Can you work these out from the model? Positions are in its coordinate system, mm. Face numbers are marked on the shaded views. A direction names the side the tool comes from. Round coordinates to 2 decimals unless told otherwise and drop trailing zeros. Loops run counter-clockwise (first coordinate to the right, second up) from the corner with the lowest first, then second, coordinate; pieces in that order, holes last. Notation, with made-up numbers: (52, 0.25) -> (92, 0.25) arc R27 cw to (92, 30.25) -> close; hole circle Ø2 at (81, 80.25). An arc over 180 degrees is marked (long way). Use a Markdown table: item, result.
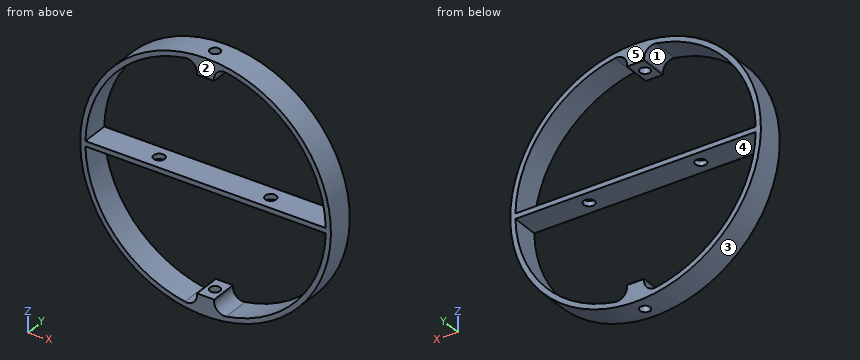
from build123d import *

# Parameters (mm, degrees)
ESQUISSE1_R             = 36.5
ESQUISSE1_R_2           = 35
BOSS_EXTRU_1_DEPTH      = 4
ENL_V_MAT_EXTRU_1_REACH = 83.714
ESQUISSE3_R             = 1.5
ENL_V_MAT_EXTRU_2_REACH = 54.305
ESQUISSE2_R             = 1.6
CONG_1_R                = 3


with BuildPart() as part:
    # Esquisse1 → Boss.-Extru.1 (new, symmetric)
    # profile 1 of 7: a face of its own
    with BuildSketch(Plane(origin=(0, 0, 0), x_dir=(1, 0, 0), z_dir=(0, 1, 0))):
        with Locations(Location((0, 0, 0), (0, 0, 270))):
            Circle(ESQUISSE1_R)
        Circle(ESQUISSE1_R_2, mode=Mode.SUBTRACT)
    # profile 2 of 7: a face of its own
    with BuildSketch(Plane(origin=(0, 0, 0), x_dir=(1, 0, 0), z_dir=(0, 1, 0))):
        with BuildLine():
            Line((34.991963363, 0.75), (0, 0.75))
            Line((0, 0.75), (0, -0.75))
            Line((0, -0.75), (34.991963363, -0.75))
            ThreePointArc((34.991963363, -0.75), (34.997990783, -0.375021529), (35, 0))
            ThreePointArc((35, 0), (34.997990783, 0.375021529), (34.991963363, 0.75))
        make_face()
    # profile 3 of 7: a face of its own
    with BuildSketch(Plane(origin=(0, 0, 0), x_dir=(1, 0, 0), z_dir=(0, 1, 0))):
        with BuildLine():
            Line((0, 0.75), (-34.991963363, 0.75))
            ThreePointArc((-34.991963363, 0.75), (-35, 0), (-34.991963363, -0.75))
            Line((-34.991963363, -0.75), (0, -0.75))
            Line((0, -0.75), (0, 0.75))
        make_face()
    # profile 4 of 7: a face of its own
    with BuildSketch(Plane(origin=(0, 0, 0), x_dir=(1, 0, 0), z_dir=(0, 1, 0))):
        with BuildLine():
            Line((0, 0.75), (-34.991963363, 0.75))
            ThreePointArc((-34.991963363, 0.75), (-35, 0), (-34.991963363, -0.75))
            Line((-34.991963363, -0.75), (0, -0.75))
            Line((0, -0.75), (0, 0.75))
        make_face()
    # profile 5 of 7: a face of its own
    with BuildSketch(Plane(origin=(0, 0, 0), x_dir=(1, 0, 0), z_dir=(0, 1, 0))):
        with BuildLine():
            Line((34.991963363, 0.75), (0, 0.75))
            Line((0, 0.75), (0, -0.75))
            Line((0, -0.75), (34.991963363, -0.75))
            ThreePointArc((34.991963363, -0.75), (34.997990783, -0.375021529), (35, 0))
            ThreePointArc((35, 0), (34.997990783, 0.375021529), (34.991963363, 0.75))
        make_face()
    # profile 6 of 7: a face of its own
    with BuildSketch(Plane(origin=(0, 0, 0), x_dir=(1, 0, 0), z_dir=(0, 1, 0))):
        with BuildLine():
            Line((-2.5, -30.910600109), (-2.5, -34.910600109))
            ThreePointArc((-2.5, -34.910600109), (0, -35), (2.5, -34.910600109))
            Line((2.5, -34.910600109), (2.5, -30.910600109))
            Line((2.5, -30.910600109), (-2.5, -30.910600109))
        make_face()
    # profile 7 of 7: a face of its own
    with BuildSketch(Plane(origin=(0, 0, 0), x_dir=(1, 0, 0), z_dir=(0, 1, 0))):
        with BuildLine():
            ThreePointArc((2.5, 34.910600109), (0, 35), (-2.5, 34.910600109))
            Line((-2.5, 34.910600109), (-2.5, 30.910600109))
            Line((-2.5, 30.910600109), (2.5, 30.910600109))
            Line((2.5, 30.910600109), (2.5, 34.910600109))
        make_face()
    extrude(amount=BOSS_EXTRU_1_DEPTH, both=True)

    # Esquisse3 → Enlèv. mat.-Extru.1 (cut, up to next)
    with BuildSketch(Plane.XY.offset(36.5), mode=Mode.PRIVATE) as enl_v_mat_extru_1_sk1:
        Circle(ESQUISSE3_R)
    enl_v_mat_extru_1_tool1 = extrude(enl_v_mat_extru_1_sk1.sketch, amount=-ENL_V_MAT_EXTRU_1_REACH, mode=Mode.PRIVATE) & part.part
    enl_v_mat_extru_1 = enl_v_mat_extru_1_tool1.solids().sort_by_distance((0, 0, 36.5))[0]
    add(enl_v_mat_extru_1, mode=Mode.SUBTRACT)

    # Symétrie1: Enlèv. mat.-Extru.1 across plane
    add(enl_v_mat_extru_1.mirror(Plane.XY), mode=Mode.SUBTRACT)

    # Esquisse2 → Enlèv. mat.-Extru.2 (cut, up to next)
    with BuildSketch(Plane.XY.offset(0.75), mode=Mode.PRIVATE) as enl_v_mat_extru_2_sk1:
        with Locations((-16.256, 0)):
            Circle(ESQUISSE2_R)
    enl_v_mat_extru_2_tool1 = extrude(enl_v_mat_extru_2_sk1.sketch, amount=-ENL_V_MAT_EXTRU_2_REACH, mode=Mode.PRIVATE) & part.part
    # Esquisse2 → Enlèv. mat.-Extru.2 (cut, up to next)
    with BuildSketch(Plane.XY.offset(0.75), mode=Mode.PRIVATE) as enl_v_mat_extru_2_sk2:
        with Locations((16.256, 0)):
            Circle(ESQUISSE2_R)
    enl_v_mat_extru_2_tool2 = extrude(enl_v_mat_extru_2_sk2.sketch, amount=-ENL_V_MAT_EXTRU_2_REACH, mode=Mode.PRIVATE) & part.part
    add(enl_v_mat_extru_2_tool1.solids().sort_by_distance((-16.256, 0, 0.75))[0], mode=Mode.SUBTRACT)
    add(enl_v_mat_extru_2_tool2.solids().sort_by_distance((16.256, 0, 0.75))[0], mode=Mode.SUBTRACT)

    # Congé1
    cong_1_edges = [part.edges().sort_by_distance(p)[0] for p in [
        (2.5, 0, -34.910600109),
        (-2.5, 0, -34.910600109),
        (-2.5, 0, 34.910600109),
        (2.5, 0, 34.910600109),
    ]]
    fillet(cong_1_edges, radius=CONG_1_R)


solid = part.part
1. If we mould it in two halves opening along Z, with no side actions, what happens to the marked faces 1, 2 and 3? For each: +Z half, -Z half, draft (parallel to the pull), parting line (faces both ways), or undercut.
Answer sheet:
| item | result |
|---|---|
| face 1 | undercut |
| face 2 | draft |
| face 3 | parting line |
2. I want a section at D-D (x = 13). Please give me the cut outline in (y, z), plus the area to 3 significant figures.
Answer sheet:
| item | result |
|---|---|
| outline | (-4, -34.11) -> (4, -34.11) -> (4, -32.5) -> (-4, -32.5) -> close; (-4, -0.75) -> (4, -0.75) -> (4, 0.75) -> (-4, 0.75) -> close; (-4, 32.5) -> (4, 32.5) -> (4, 34.11) -> (-4, 34.11) -> close |
| area | 37.8 mm² |
3. I need wall thicknesses on line 1 (Z direction, x = -27, y = -3.25); line 2 (Z direction, x = 16.5, y = -2); line 3 (Y direction, x = 0, z = 34.7). Which ranges of each line are inside material? Lowest first, please.
Answer sheet:
| item | result |
|---|---|
| line 1 | z = -24.56 to -22.27, -0.75 to 0.75, 22.27 to 24.56 |
| line 2 | z = -32.56 to -30.87, -0.75 to 0.75, 30.87 to 32.56 |
| line 3 | y = -4 to -1.5, 1.5 to 4 |
4. I want a section at B-B (y = 2.75). Please give me the cut outline in (x, z), plus the area to 3 significant figures.
Answer sheet:
| item | result |
|---|---|
| outline | circle Ø73 at (0, 0); hole (-34.99, -0.75) arc R35 ccw to (-6.02, -34.48) arc R3 ccw to (-2.5, -31.52) -> (-2.5, -30.91) -> (2.5, -30.91) -> (2.5, -31.52) arc R3 ccw to (6.02, -34.48) arc R35 ccw to (34.99, -0.75) -> close; hole (-34.99, 0.75) -> (34.99, 0.75) arc R35 ccw to (6.02, 34.48) arc R3 ccw to (2.5, 31.52) -> (2.5, 30.91) -> (-2.5, 30.91) -> (-2.5, 31.52) arc R3 ccw to (-6.02, 34.48) arc R35 ccw to start |
| area | 493 mm² |
5. Will these pins go through, and if not, where does the flat tip stop? pin 1 Ø3.5 at (x, y) = (16.256, 0) entering from -Z; pin 2 Ø2.5 at (x, y) = (0, 0) entering from -Z; pin 3 Ø0.7 at (y, z) = (2, 31.5) entering from -X; pin 4 Ø4 at (x, y) = (0, 0) entering from -Z.
Answer sheet:
| item | result |
|---|---|
| pin 1 | stops at z = -33.49 |
| pin 2 | stops at z = -0.75 |
| pin 3 | stops at x = -19.02 |
| pin 4 | stops at z = -36.5 |
6. I want a section at C-C (z = 4.5). Please give me the cut outline in (x, y), plus the area to 3 significant figures.
Answer sheet:
| item | result |
|---|---|
| outline | (-36.22, -4) -> (-34.71, -4) -> (-34.71, 4) -> (-36.22, 4) -> close; (34.71, -4) -> (36.22, -4) -> (36.22, 4) -> (34.71, 4) -> close |
| area | 24.2 mm² |
7. I want a section at A-A (x = 0). Please give me the cut outline in (y, z).
Answer sheet:
| item | result |
|---|---|
| outline | (-4, -36.5) -> (-1.5, -36.5) -> (-1.5, -30.91) -> (-4, -30.91) -> close; (-4, -0.75) -> (4, -0.75) -> (4, 0.75) -> (-4, 0.75) -> close; (-4, 30.91) -> (-1.5, 30.91) -> (-1.5, 36.5) -> (-4, 36.5) -> close; (1.5, -36.5) -> (4, -36.5) -> (4, -30.91) -> (1.5, -30.91) -> close; (1.5, 30.91) -> (4, 30.91) -> (4, 36.5) -> (1.5, 36.5) -> close |
8. Which directions (+Z, -Z, +X, -X, +Y, -Y) give clear straight access to the entire face, cutting with the end or side of a thin tool? Please do the marked faces 4 and 5.
Answer sheet:
| item | result |
|---|---|
| face 4 | +Y, -Y |
| face 5 | +Z, -Z, +X, -X, +Y |
